Verification items for the finished model (mm, model axes). A direction names the side the tool comes from. Give positions to 0.01 mm unless a question says otherwise; leave off trailing zeros. Order: outer loops, then holes, each group sorted by start corner. A loop starts at its lowest first (then second) coordinate and runs counter-clockwise, first axis right, second up. Notation, with made-up numbers: (-9.5, 20.25) -> (39.5, 20.25) arc R24 cw to (39.5, 30.25) -> close; hole circle Ø6 at (-37, -10.5). An arc over 180 degrees is marked (long way). Return JSON: item names as keys, results as strings. Group by question number.
(1) Tool access check on faces 1 (the face through (2.799, -6.907, 3.905)), 2 (the face through (-3, 5, 10.129)), 3 (the face through (5.723, -1.802, 12.157)). Record the directions out of +Z, -Z, +X, -X, +Y, -Y that give a thin tool (end or side, any length) a straight path to the whole face; none if there is none.
(2) Release check for a two-part mould opening along X. For faces 4 (the face through (-7, 1.6, 5.4)), 5 (the face through (4.9, 2, 4.4)), 6 (the face through (7, 7, 2)) record: pulls with the +X half, pulls with the -X half, needs draft (parallel to the pull), parting line crosses it, or undercut.
(3) Cross-section at A-A on y = 14.5. Enter the section's corners in (x, z).
(4) Thickness scan on line 1 along Z through (x, y) = (4.5, -17); line 2 along Y through (x, z) = (1.5, 9.75); line 3 along X through (y, z) = (-29, 1.2). Record the ranges inside material, lowest first.
(5) Cross-section at C-C on y = 29. Enter the section's corners in (x, z), then the cut area to 3 significant figures.
(6) Cross-section at D-D on z = 11.75. Enter the section's corners in (x, y).
(7) Depth check by flat-ended pin: pin 1 Ø2.5 at (y, z) = (3, 4.5) entering from -X; pin 2 Ø2.5 at (y, z) = (2.5, 4.5) entering from +X; pin 3 Ø2.5 at (x, y) = (0.5, 0) entering from +Z; pin 4 Ø0.6 at (x, y) = (6.5, 4.5) entering from +Z. Enter the tip coordinate at first touch or a pass-through.
(8) Cross-section at B-B on z = 4.5. Enter the section's corners in (x, y) (3 decimals), then the cut area to 3 significant figures.
from build123d import *
from OCP.BRepFilletAPI import BRepFilletAPI_MakeChamfer

# Parameters (mm, degrees)
F_6_5_6_5_DIAMETER_HOLE1_D   = 6.5
F_7_0_7_DIAMETER_HOLE1_D     = 7
F_7_0_7_DIAMETER_HOLE1_DEPTH = 9
F_7_0_7_DIAMETER_HOLE1_TIP   = 2.103012167
DRILL_START                  = -7
DRILL_FLAT_DEPTH             = 42.01171732
FUEL_INLET_REACH             = 54.902
FUEL_INLET_END_RADIUS        = 3.25
SKETCH7_R                    = 0.75
INLETS_COUNT                 = 3
SKETCH10_W                   = 1
SKETCH10_H                   = 0.5
TOOL_RAD_R                   = 0.5
EDGE_BREAK_SIZE              = 0.25
EDGE_BREAK_SIZE2             = 0.683012702
F_2_2_2_2_DIAMETER_HOLE1_D   = 2.2
CIRPATTERN1_COUNT            = 6


with BuildPart() as part:
    # Sketch2 → Main Base (revolve)
    with BuildSketch(Plane(origin=(0, 0, 0), x_dir=(0, 0, -1), z_dir=(1, 0, 0)), mode=Mode.PRIVATE) as main_base_sk:
        Polygon((0, 0), (0, 31.75), (-2, 31.75), (-2, 8), (-7, 8), (-7, 6), (-17, 6), (-17, 0), align=None)
    revolve(main_base_sk.sketch.rotate(Axis((0, 0, -29.195597269), (0, 0, -1)), 90), axis=Axis((0, 0, -29.195597269), (0, 0, -1)))

    # Ø6.5 (6.5) Diameter Hole1 (through all)
    with Locations(Plane.XY.offset(17)):
        with Locations((0, 0)):
            Hole(F_6_5_6_5_DIAMETER_HOLE1_D / 2)

    # Ø7.0 (7) Diameter Hole1
    with Locations(Plane.XY.offset(17)):
        with Locations((0, 0)):
            Hole(F_7_0_7_DIAMETER_HOLE1_D / 2, depth=F_7_0_7_DIAMETER_HOLE1_DEPTH)
            with Locations((0, 0, -(F_7_0_7_DIAMETER_HOLE1_DEPTH + F_7_0_7_DIAMETER_HOLE1_TIP / 2))):  # 118° drill point
                Cone(0, F_7_0_7_DIAMETER_HOLE1_D / 2, F_7_0_7_DIAMETER_HOLE1_TIP, mode=Mode.SUBTRACT)

    # Sketch6 → Drill Flat (cut, through all)
    with BuildSketch(Plane(origin=(0, 0, 0), x_dir=(0, 0, -1), z_dir=(1, 0, 0)).offset(DRILL_START)):
        with BuildLine():
            Line((-6.175, 0.075), (-7, 0.075))
            ThreePointArc((-7, 0.075), (-9.24506403, 1.00493597), (-10.175, 3.25))
            Line((-10.175, 3.25), (-10.175, 8))
            Line((-10.175, 8), (-3, 8))
            Line((-3, 8), (-3, 3.25))
            ThreePointArc((-3, 3.25), (-3.92993597, 1.00493597), (-6.175, 0.075))
        make_face()
    drill_flat = extrude(amount=-DRILL_FLAT_DEPTH, mode=Mode.SUBTRACT)

    # Fuel Inlet: up to this cylinder (the profile starts outside it)
    fuel_inlet_end = Plane(origin=(0, 0, 4.5), z_dir=(0, 0, 1)) * Cylinder(FUEL_INLET_END_RADIUS, 117.304, mode=Mode.PRIVATE)
    # Sketch7 → Fuel Inlet (cut, up to the surface)
    with BuildSketch(Plane.ZY.offset(7), mode=Mode.PRIVATE) as fuel_inlet_sk1:
        with Locations((4.5, 2.5)):
            Circle(SKETCH7_R)
    fuel_inlet_tool1 = extrude(fuel_inlet_sk1.sketch, amount=-FUEL_INLET_REACH, mode=Mode.PRIVATE) - fuel_inlet_end
    fuel_inlet = fuel_inlet_tool1.solids().sort_by_distance((-7, 2.5, 4.5))[0]
    add(fuel_inlet, mode=Mode.SUBTRACT)

    # Inlets: Drill Flat, Fuel Inlet ×3 about axis
    inlets_axis = Axis((0, 0, 0), (0, 0, 1))
    add([drill_flat.rotate(inlets_axis, i * 360 / INLETS_COUNT) for i in range(1, INLETS_COUNT)], mode=Mode.SUBTRACT)
    add([fuel_inlet.rotate(inlets_axis, i * 360 / INLETS_COUNT) for i in range(1, INLETS_COUNT)], mode=Mode.SUBTRACT)

    # Sketch8 → Cone Cut (revolve, cut)
    with BuildSketch(Plane(origin=(0, 0, 0), x_dir=(0, 0, -1), z_dir=(1, 0, 0)), mode=Mode.PRIVATE) as cone_cut_sk:
        Polygon((-7, 6), (-5.845299462, 8), (-7, 8), align=None)
    revolve(cone_cut_sk.sketch.rotate(Axis((0, 0, 58.5), (0, 0, -1)), 90), axis=Axis((0, 0, 58.5), (0, 0, -1)), mode=Mode.SUBTRACT)

    # Sketch10 → Radial O-rings (revolve, cut)
    with BuildSketch(Plane(origin=(0, 0, 0), x_dir=(0, 0, -1), z_dir=(1, 0, 0)), mode=Mode.PRIVATE) as radial_o_rings_sk:
        with Locations((-9.628768748, 5.75)):
            Rectangle(SKETCH10_W, SKETCH10_H)
        with Locations((-14.628768748, 5.75)):
            Rectangle(SKETCH10_W, SKETCH10_H)
    revolve(radial_o_rings_sk.sketch.rotate(Axis((0, 0, 58.5), (0, 0, -1)), 90), axis=Axis((0, 0, 58.5), (0, 0, -1)), mode=Mode.SUBTRACT)

    # Sketch11 → ORB Port (revolve, cut)
    with BuildSketch(Plane(origin=(0, 0, 0), x_dir=(0, 0, -1), z_dir=(1, 0, 0)), mode=Mode.PRIVATE) as orb_port_sk:
        Polygon((-17, 4.55), (-14.8, 4.082375564), (-14.8, 3.5), (-17, 3.5), align=None)
    revolve(orb_port_sk.sketch.rotate(Axis((0, 0, 17.730420959), (0, 0, -1)), 90), axis=Axis((0, 0, 17.730420959), (0, 0, -1)), mode=Mode.SUBTRACT)

    # Tool Rad
    tool_rad_edges = [part.edges().sort_by_distance(p)[0] for p in [
        (-6, 0, 7),
        (-8, 0, 2),
    ]]
    fillet(tool_rad_edges, radius=TOOL_RAD_R)

    # Edge Break: one chamfer whose edges measure the first distance from different faces: ONE call of the kernel's chamfer builder (chamfer() names one face for all edges)
    edge_break_edges_1 = [part.edges().sort_by_distance(p)[0] for p in [
        (-6, 0, 17),
        (5.665063509, 4.812177826, 3.75),
        (1.334936491, -7.312177826, 3.75),
        (-7, 2.5, 3.75),
    ]]
    edge_break_edges_2 = [part.edges().sort_by_distance(p)[0] for p in [
        (-5.637822703, -5.675821982, 5.845299462),
        (-2.096494672, 7.720408674, 5.845299462),
        (6.905046679, -4.039842864, 5.845299462),
    ]]
    edge_break_side_2 = [part.faces().sort_by_distance(p)[0] for p in [
        (-8, 0, 4.172649731),
    ]]
    edge_break = BRepFilletAPI_MakeChamfer(part.part.solid().wrapped)
    for e in edge_break_edges_1:
        edge_break.Add(EDGE_BREAK_SIZE, e.wrapped)
    for e in edge_break_edges_2:
        edge_break.Add(EDGE_BREAK_SIZE, EDGE_BREAK_SIZE2, e.wrapped, edge_break_side_2[0].wrapped)  # the first distance lies on this face
    add(Compound.cast(edge_break.Shape()), mode=Mode.REPLACE)

    # Ø2.2 (2.2) Diameter Hole1 (through all)
    with Locations(Plane.XY.offset(2)):
        with Locations((0, 29)):
            f_2_2_2_2_diameter_hole1 = Hole(F_2_2_2_2_DIAMETER_HOLE1_D / 2)

    # CirPattern1: Ø2.2 (2.2) Diameter Hole1 ×6 about axis
    cirpattern1_axis = Axis((0, 0, 0), (0, 0, 1))
    for i in range(1, CIRPATTERN1_COUNT):
        add(f_2_2_2_2_diameter_hole1.rotate(cirpattern1_axis, i * 360 / CIRPATTERN1_COUNT), mode=Mode.SUBTRACT)


solid = part.part
Verdict:
{
 "1": {"face 1": "+Z, -Y", "face 2": "none", "face 3": "+Z"},
 "2": {"face 4": "pulls with the -X half", "face 5": "undercut", "face 6": "needs draft"},
 "3": {"outline": "(-28.25, 0) -> (-26.21, 0) -> (-26.21, 2) -> (-28.25, 2) -> close; (-24.01, 0) -> (24.01, 0) -> (24.01, 2) -> (-24.01, 2) -> close; (26.21, 0) -> (28.25, 0) -> (28.25, 2) -> (26.21, 2) -> close"},
 "4": {"line 1": "0 to 2", "line 2": "-5.29 to -3.16, 3.16 to 5.29", "line 3": "-12.93 to -1.1, 1.1 to 12.93"},
 "5": {"outline": "(-12.93, 0) -> (-1.1, 0) -> (-1.1, 2) -> (-12.93, 2) -> close; (1.1, 0) -> (12.93, 0) -> (12.93, 2) -> (1.1, 2) -> close", "area": "47.3 mm²"},
 "6": {"outline": "circle Ø12 at (0, 0); hole circle Ø7 at (0, 0)"},
 "7": {"pin 1": "x = -7", "pin 2": "x = 7.9", "pin 3": "through", "pin 4": "z = 5.99"},
 "8": {"outline": "(-7.981, 0.553) arc R8 ccw to (0.146, -7.999) -> (0.469, -7.812) -> (0.56, -7.471) -> (-2.815, -1.625) arc R3.25 cw to (-2.739, 1.75) -> (-6.75, 1.75) -> (-7, 1.5) -> (-7, 0.553) -> close; (-7, 3.5) -> (-6.75, 3.25) -> (0, 3.25) arc R3.25 cw to (2.885, 1.497) -> (4.891, 4.971) -> (4.799, 5.312) -> (3.979, 5.786) -> (4.469, 6.635) arc R8 ccw to (-7, 3.873) -> close; (-0.146, -3.247) -> (1.859, -6.721) -> (2.201, -6.812) -> (3.021, -6.339) -> (3.512, -7.188) arc R8 ccw to (6.854, 4.126) -> (6.531, 4.312) -> (6.19, 4.221) -> (2.815, -1.625) arc R3.25 cw to start", "area": "139 mm²"}
}
